Autodesk Fusion 360 part; units mm, degrees
sketch "Sketch1" plane through (0, 0, 0) normal (0, 0, 1) x (1, 0, 0)
  line L0 (-80, 100) -> (80, 100)
  line L1 (100, 80) -> (100, -80)
  line L2 (80, -100) -> (-80, -100)
  line L3 (-100, -80) -> (-100, 80)
  line L4 (-80, 100) -> (-100, 80)
  line L5 (80, 100) -> (100, 80)
  line L6 (-80, -100) -> (-100, -80)
  line L7 (100, -80) -> (80, -100)
  circle A0 centre (90, 80) radius 2.5
  circle A1 centre (80, 90) radius 2.5
  circle A2 centre (-81.762, 90) radius 2.5
  circle A3 centre (-90, 80) radius 2.5
  circle A4 centre (-90, -80) radius 2.5
  circle A5 centre (-80, -90) radius 2.5
  circle A6 centre (75, -90) radius 2.5
  circle A7 centre (90, -80) radius 2.5
  point P0 (-100, 100)
  point P1 (100, 100)
  point P2 (100, -100)
  point P3 (-100, -100)
  dimension "d4" = 200
  dimension "d5" = 200
  dimension "d6" = 20
  dimension "d7" = 20
  dimension "d8" = 20
  dimension "d9" = 20
  dimension "d10" = 20
  dimension "d11" = 20
  dimension "d12" = 20
  dimension "d13" = 20
  dimension "d14" = 5
  dimension "d15" = 5
  dimension "d16" = 5
  dimension "d17" = 5
  dimension "d18" = 5
  dimension "d19" = 5
  dimension "d20" = 5
  dimension "d21" = 5
extrude "Extrude2" add sketch "Sketch1" along normal blind 10
extrude "Extrude1" [suppressed]
equation "d7 = d6"
equation "d9 = d8"
equation "d11 = d10"
equation "d13 = d12"
Model file for the job. Use its own axes, mm. Round coordinates to 2 decimals unless told otherwise and drop trailing zeros. Loops run counter-clockwise (first coordinate to the right, second up) from the corner with the lowest first, then second, coordinate; pieces in that order, holes last.
1. Mould opens along Y. For faces 1 (the cylindrical face through (87.5, 79.9, 4.9)), 2 (the cylindrical face through (79.67, 87.52, 4.93)), 3 (the flat face through (100, 1, 5)), 4 (the flat face through (-90, -90, 5)) say: +Y half, -Y half, draft (parallel to the pull), parting line (faces both ways), or undercut.
Check values:
face 1: undercut
face 2: undercut
face 3: draft
face 4: -Y half
2. Drop a flat-ended pin along its axis: P1, Ø4.5, axis at x = 75, y = -90, coming from the +Z side. Give the stop position or say it passes through.
Check values:
P1: passes through
3. Band-saw the part on B-B, the plane x = 75. List the corners of the cut face in (y, z).
Check values:
outline: (-100, 0) - (-92.5, 0) - (-92.5, 10) - (-100, 10) - close; (-87.5, 0) - (100, 0) - (100, 10) - (-87.5, 10) - close
4. Band-saw the part on C-C, the plane z = 1.75. Count the separate pieces of the cut face and the enclosed holes in it, and give its area (3 significant figures).
Check values:
separate pieces: 1
enclosed holes: 8
area: 39,000 mm2
5. Wall check: probe 1 along Y at (x, z) = (80, 8); probe 2 along Y at (x, z) = (75, 8.25); probe 3 along Y at (x, z) = (-80, 2.25). Give the ranges that are in metal, low to high.
Check values:
probe 1: y = -100 to 87.5, 92.5 to 100
probe 2: y = -100 to -92.5, -87.5 to 100
probe 3: y = -100 to -92.5, -87.5 to 88.23, 91.77 to 100
6. Band-saw the part on A-A, the plane y = -90. List the corners of the cut face in (x, z).
Check values:
outline: (-90, 0) - (-82.5, 0) - (-82.5, 10) - (-90, 10) - close; (-77.5, 0) - (72.5, 0) - (72.5, 10) - (-77.5, 10) - close; (77.5, 0) - (90, 0) - (90, 10) - (77.5, 10) - close
